Check sheet for the drawn part. Datum: minimum x, y, z corner. Units: mm. A direction names the side the tool comes from. Round coordinates to 2 decimals unless told otherwise and drop trailing zeros. Write each loop counter-clockwise with the first axis right and the second up, starting at its lowest first coordinate (ties: lowest second). Pieces come first, ordered by that corner, then holes. Notation, with made-up numbers: (28.25, 42.25) -> (71.25, 42.25) arc R10 cw to (71.25, 51.25) -> close; hole circle Ø7 at (45.5, 40). An arc over 180 degrees is marked (long way). Use a Markdown table: item, result.
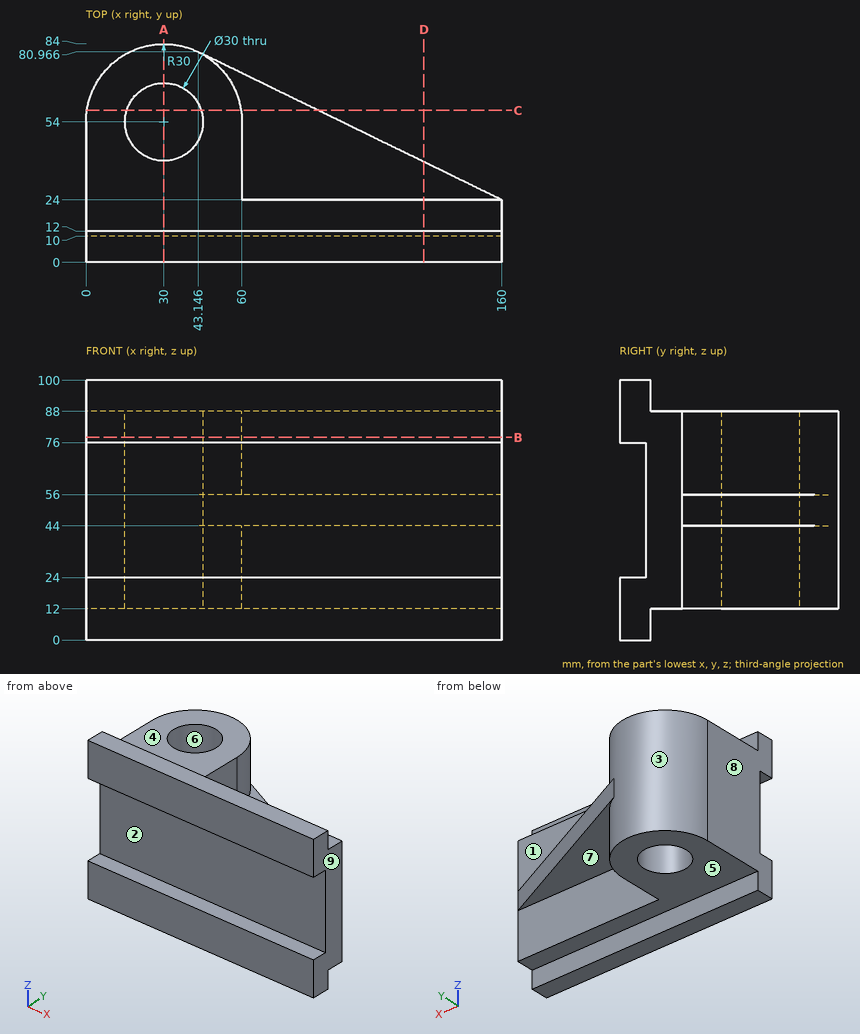
(1) Section check B-B on z = 78. Record the cut outline in (x, y), plus the area to 3 significant figures.
A:
| item | result |
|---|---|
| outline | (0, 0) -> (160, 0) -> (160, 24) -> (60, 24) -> (60, 54) arc R30 ccw to (0, 54) -> close; hole circle Ø30 at (30, 54) |
| area | 6,350 mm2 |
(2) Access from +Z, -Z, +X, -X, +Y, -Y to the whole of each face (thin tool, end or side, straight path). Record for the marked faces 1, 2, 3, 4 and 5.
A:
| item | result |
|---|---|
| face 1 | +Z, +X, +Y |
| face 2 | +X, -X, -Y |
| face 3 | +Y |
| face 4 | +Z, +X, -X, +Y |
| face 5 | -Z, +X, -X, +Y |
(3) Section check D-D on x = 130. Record the cut outline in (y, z) (1 decimal), plus the area to 3 significant figures.
A:
| item | result |
|---|---|
| outline | (0, 0) -> (12, 0) -> (12, 12) -> (24, 12) -> (24, 44) -> (38.6, 44) -> (38.6, 56) -> (24, 56) -> (24, 88) -> (12, 88) -> (12, 100) -> (0, 100) -> (0, 76) -> (10, 76) -> (10, 24) -> (0, 24) -> close |
| area | 1,770 mm2 |
(4) Thickness scan on line 1 (Y direction, x = 30, z = 31); line 2 (Z direction, x = 140, y = 7); line 3 (X direction, y = 35.5, z = 60). Record the ranges inside material, lowest first.
A:
| item | result |
|---|---|
| line 1 | y = 10 to 39, 69 to 84 |
| line 2 | z = 0 to 24, 76 to 100 |
| line 3 | x = 0 to 60 |
(5) Section check C-C on y = 58.5. Record the cut outline in (x, z).
A:
| item | result |
|---|---|
| outline | (0.34, 12) -> (15.69, 12) -> (15.69, 88) -> (0.34, 88) -> close; (44.31, 12) -> (59.66, 12) -> (59.66, 44) -> (89.23, 44) -> (89.23, 56) -> (59.66, 56) -> (59.66, 88) -> (44.31, 88) -> close |
(6) Section check A-A on x = 30. Record the cut outline in (y, z).
A:
| item | result |
|---|---|
| outline | (0, 0) -> (12, 0) -> (12, 12) -> (39, 12) -> (39, 88) -> (12, 88) -> (12, 100) -> (0, 100) -> (0, 76) -> (10, 76) -> (10, 24) -> (0, 24) -> close; (69, 12) -> (84, 12) -> (84, 88) -> (69, 88) -> close |
(7) Gauge pin test, flat ends, axial feed: pin 1 Ø24 at (y, z) = (45, 71.5) entering from +X; pin 2 Ø2 at (x, z) = (90, 71.5) entering from +Y; pin 3 Ø3.5 at (x, z) = (82, 92.5) entering from +Y. Record the tip position at first contact, or that the pin passes through.
A:
| item | result |
|---|---|
| pin 1 | stops at x = 60 |
| pin 2 | stops at y = 24 |
| pin 3 | stops at y = 12 |
(8) Release check for a two-part mould opening along X. For the marked faces 6, 7, 8 and 9 record: +X half, -X half, draft (parallel to the pull), parting line (faces both ways), or undercut.
A:
| item | result |
|---|---|
| face 6 | undercut |
| face 7 | draft |
| face 8 | -X half |
| face 9 | +X half |
